```python
from build123d import *

# Parameters (mm, degrees)
SKETCH1_W               = 101.6
SKETCH1_H               = 57.15
BOSS_EXTRUDE1_DEPTH     = 3.175
SKETCH10_R              = 1.5
CUT_EXTRUDE3_DEPTH      = 59.371664787
FILLET1_R               = 2.54
CUT_EXTRUDE4_DEPTH      = 59.371664787
CUT_EXTRUDE4_DEPTH_BACK = 59.371664787
SKETCH12_R              = 2.794
BOSS_EXTRUDE3_DEPTH     = 1.397
SKETCH13_R              = 2.794
BOSS_EXTRUDE4_DEPTH     = 1.397
FILLET4_R               = 1
SKETCH14_W              = 50.8
SKETCH14_H              = 5.9817
SKETCH14_W_2            = 19.058479039
SKETCH14_W_3            = 6.2611
SKETCH14_H_2            = 19.7866
SKETCH14_H_3            = 5.715
BOSS_EXTRUDE5_DEPTH     = 11.176
SKETCH15_W              = 3.2131
SKETCH15_H              = 19.7866
SKETCH15_W_2            = 19.058479039
SKETCH15_H_2            = 2.9337
SKETCH15_H_3            = 5.715
SKETCH15_W_3            = 50.8
BOSS_EXTRUDE6_DEPTH     = 3.048


with BuildPart() as part:
    # Sketch1 → Boss-Extrude1 (new body)
    with BuildSketch(Plane(origin=(0, 0, 0), x_dir=(1, 0, 0), z_dir=(0, 1, 0))):
        Rectangle(SKETCH1_W, SKETCH1_H)
    extrude(amount=BOSS_EXTRUDE1_DEPTH)

    # Sketch10 → Cut-Extrude3 (cut, through all)
    with BuildSketch(Plane(origin=(0, 3.175, 0), x_dir=(1, 0, 0), z_dir=(0, 1, 0))):
        with Locations(Location((-45.212, -22.987, 0), (0, 0, 270))):
            Circle(SKETCH10_R)
        with Locations(Location((45.212, 22.987, 0), (0, 0, 270))):
            Circle(SKETCH10_R)
        with Locations(Location((-45.212, 22.987, 0), (0, 0, 270))):
            Circle(SKETCH10_R)
        with Locations(Location((45.212, -22.987, 0), (0, 0, 270))):
            Circle(SKETCH10_R)
    extrude(amount=-CUT_EXTRUDE3_DEPTH, mode=Mode.SUBTRACT)

    # Fillet1
    fillet1_edges = [part.edges().sort_by_distance(p)[0] for p in [
        (-50.8, 1.5875, -28.575),
        (50.8, 1.5875, -28.575),
        (50.8, 1.5875, 28.575),
        (-50.8, 1.5875, 28.575),
    ]]
    fillet(fillet1_edges, radius=FILLET1_R)

    # Sketch11 → Cut-Extrude4 (cut, two sides: drawn at the far end of the back side and taken through both)
    with BuildSketch(Plane(origin=(0, 3.175, 0), x_dir=(1, 0, 0), z_dir=(0, 1, 0)).offset(-CUT_EXTRUDE4_DEPTH_BACK)):
        with BuildLine():
            Line((-33.224345588, 18.800272814), (7.451171928, 18.800272814))
            ThreePointArc((7.451171928, 18.800272814), (10.626171928, 15.625272814), (7.451171928, 12.450272814))
            Line((7.451171928, 12.450272814), (-33.224345588, 12.450272814))
            ThreePointArc((-33.224345588, 12.450272814), (-36.399345588, 15.625272814), (-33.224345588, 18.800272814))
        make_face()
    extrude(amount=CUT_EXTRUDE4_DEPTH + CUT_EXTRUDE4_DEPTH_BACK, mode=Mode.SUBTRACT)

    # Sketch12 → Boss-Extrude3 (add, symmetric)
    with BuildSketch(Plane(origin=(2.9972, 0, 0), x_dir=(0, 0, -1), z_dir=(1, 0, 0))):
        with BuildLine():
            Line((-7.5057, 0), (7.5057, 0))
            Line((7.5057, 0), (10.6807, 0))
            Line((10.6807, 0), (7.5057, -8.0518))
            ThreePointArc((7.5057, -8.0518), (0, -15.5575), (-7.5057, -8.0518))
            Line((-7.5057, -8.0518), (-10.6807, 0))
            Line((-10.6807, 0), (-7.5057, 0))
        make_face()
        with Locations((0, -8.0518)):
            Circle(SKETCH12_R, mode=Mode.SUBTRACT)
    extrude(amount=BOSS_EXTRUDE3_DEPTH, both=True)

    # Sketch13 → Boss-Extrude4 (add, symmetric)
    with BuildSketch(Plane(origin=(-2.9972, 0, 0), x_dir=(0, 0, -1), z_dir=(1, 0, 0))):
        with BuildLine():
            Line((-7.5057, 0), (7.5057, 0))
            Line((7.5057, 0), (10.6807, 0))
            Line((10.6807, 0), (7.5057, -8.0518))
            ThreePointArc((7.5057, -8.0518), (0, -15.5575), (-7.5057, -8.0518))
            Line((-7.5057, -8.0518), (-10.6807, 0))
            Line((-10.6807, 0), (-7.5057, 0))
        make_face()
        with Locations((0, -8.0518)):
            Circle(SKETCH13_R, mode=Mode.SUBTRACT)
    extrude(amount=BOSS_EXTRUDE4_DEPTH, both=True)

    # Fillet4
    fillet4_edges = [part.edges().sort_by_distance(p)[0] for p in [
        (4.3942, 0, 0),
        (2.9972, -8.0518, 7.5057),
        (2.9972, -8.0518, -7.5057),
        (1.6002, 0, 0),
        (2.9972, 0, -10.6807),
        (2.9972, 0, 10.6807),
        (-1.6002, 0, 0),
        (-2.9972, 0, 10.6807),
        (-2.9972, -8.0518, 7.5057),
        (-2.9972, -8.0518, -7.5057),
        (-4.3942, 0, 0),
        (-2.9972, 0, -10.6807),
    ]]
    fillet(fillet4_edges, radius=FILLET4_R)

    # Sketch14 → Boss-Extrude5 (add)
    with BuildSketch(Plane(origin=(0, 3.175, 0), x_dir=(1, 0, 0), z_dir=(0, 1, 0))):
        with Locations((-10.8331, -18.47215)):
            Rectangle(SKETCH14_W, SKETCH14_H)
        with Locations((25.870411448, 18.47215)):
            Rectangle(SKETCH14_W_2, SKETCH14_H)
        with Locations((40.55745, 0)):
            Rectangle(SKETCH14_W_3, SKETCH14_H_2)
        with Locations((-40.55745, 10.7188)):
            Rectangle(SKETCH14_W_3, SKETCH14_H_3)
    extrude(amount=BOSS_EXTRUDE5_DEPTH)

    # Sketch15 → Boss-Extrude6 (add)
    with BuildSketch(Plane(origin=(0, 14.351, 0), x_dir=(1, 0, 0), z_dir=(0, 1, 0))):
        with Locations((42.08145, 0)):
            Rectangle(SKETCH15_W, SKETCH15_H)
        with Locations((25.870411448, 19.99615)):
            Rectangle(SKETCH15_W_2, SKETCH15_H_2)
        with Locations((-42.08145, 10.7188)):
            Rectangle(SKETCH15_W, SKETCH15_H_3)
        with Locations((-10.8331, -19.99615)):
            Rectangle(SKETCH15_W_3, SKETCH15_H_2)
    extrude(amount=BOSS_EXTRUDE6_DEPTH)


solid = part.part
```
The listing builds one solid part. Answer for the finished solid, in the listing's coordinates (mm). A direction names the side the tool comes from. Give positions to 0.01 mm unless a question says otherwise; leave off trailing zeros. Loops run counter-clockwise (first coordinate to the right, second up) from the corner with the lowest first, then second, coordinate; pieces in that order, holes last. Notation, with made-up numbers: (57, 8.25) - (112, 8.25) arc R6 ccw to (112, 16.25) - close; hole circle Ø2 at (75.5, 5.25). An arc over 180 degrees is marked (long way). Return JSON: item names as keys, results as strings. Group by question number.
1. Determine the mould class of faces 5 (the cylindrical face through (-50.076, 1.61, 27.811)), 6 (the flat face through (3.02, -4.31, 8.98)), 7 (the cylindrical face through (-3.02, -5.28, 0.36)) for opening direction Y: pulls with the +Y half, pulls with the -Y half, needs draft (parallel to the pull), parting line crosses it, or undercut.
2. Find section A-A (z = 0). State how many separate pieces and enclosed holes the cut face has, then the cut area to 3 significant figures.
3. Find section C-C (x = 24.5). Write down the section's boundary in (y, z) (3 decimals), then the cut area to 3 significant figures.
4. Given pin 1 Ø0.9 at (x, z) = (-13.5, 17.5) entering from +Y; pin 2 Ø1.5 at (x, y) = (27.5, 15.5) entering from +Z; pin 3 Ø3 at (y, z) = (7.5, -17) entering from -X, each flat-ended and moving along its own axis, determine where each tip first touches the part or whether it passes through.
5. Find section D-D (x = 8.5). Write down the section's boundary in (y, z) (3 decimals), then the cut area to 3 significant figures.
6. Which of the six approach directions +Z, -Z, +X, -X, +Y, -Y give full straight-line access (tool end or side, diameter ignored) to faces 1 (the cylindrical face through (10.625, 1.565, -15.695)), 2 (the flat face through (-37.427, 9, -11)), 3 (the flat face through (26, 10, -21.463)), 4 (the flat face through (-4.394, -5, 0))?
7. Find section B-B (y = 8). Write down the section's boundary in (x, z), then the cut area to 3 significant figures.
8. Straight lines are drawn through the part: line 1 (Y direction, x = 26, z = 2) (3 decimals); line 2 (Y direction, x = -28, z = 19.5); line 3 (Z direction, x = -29, y = 12). For each, find the intervals that lie inside material, in ascending order. Write a range as [from, to].
Verdict:
{
 "1": {"face 5": "needs draft", "face 6": "pulls with the -Y half", "face 7": "undercut"},
 "2": {"separate pieces": "3", "enclosed holes": "0", "area": "459 mm^2"},
 "3": {"outline": "(0, -28.575) - (3.175, -28.575) - (3.175, -21.463) - (17.399, -21.463) - (17.399, -18.529) - (14.351, -18.529) - (14.351, -15.481) - (3.175, -15.481) - (3.175, 28.575) - (0, 28.575) - close", "area": "257 mm^2"},
 "4": {"pin 1": "stops at y = 14.35", "pin 2": "stops at z = -18.53", "pin 3": "stops at x = 16.34"},
 "5": {"outline": "(0, -28.575) - (3.175, -28.575) - (3.175, -18.622) - (0, -18.622) - close; (0, -12.629) - (3.175, -12.629) - (3.175, 15.481) - (14.351, 15.481) - (14.351, 18.529) - (17.399, 18.529) - (17.399, 21.463) - (3.175, 21.463) - (3.175, 28.575) - (0, 28.575) - close", "area": "238 mm^2"},
 "6": {"face 1": "+Y, -Y", "face 2": "+Z, -Z, +Y", "face 3": "-Z, +X, -X, +Y", "face 4": "+Z, -Z, -X, -Y"},
 "7": {"outline": "(-43.69, -13.58) - (-37.43, -13.58) - (-37.43, -7.86) - (-43.69, -7.86) - close; (-36.23, 15.48) - (14.57, 15.48) - (14.57, 21.46) - (-36.23, 21.46) - close; (16.34, -21.46) - (35.4, -21.46) - (35.4, -15.48) - (16.34, -15.48) - close; (37.43, -9.89) - (43.69, -9.89) - (43.69, 9.89) - (37.43, 9.89) - close", "area": "578 mm^2"},
 "8": {"line 1": "y = [0, 3.175]", "line 2": "y = [0, 17.4]", "line 3": "z = [15.48, 21.46]"}
}
